from build123d import *

# Parameters (mm, degrees)
F0_W     = 25.908
F0_H     = 5.08
F1_DEPTH = 3.048
F2_W     = 25.908
F2_H     = 3.048
F3_DEPTH = 28.448
F4_R     = 0.762
F4_R_2   = 1.27
F5_DEPTH = 25.4
F6_R     = 1.778
F7_DEPTH = 25.4
F8_DEPTH = 2.032


with BuildPart() as f1:
    # F0 (on Top) → F1 (new body)
    with BuildSketch(Plane.XY):
        Rectangle(F0_W, F0_H)
    extrude(amount=F1_DEPTH)

    # F2 (on face) → F3 (join)
    with BuildSketch(Plane(origin=(0, 0, 0), x_dir=(1, 0, 0), z_dir=(0, 0, -1))):
        with Locations((0, 4.064)):
            Rectangle(F2_W, F2_H)
    extrude(amount=-F3_DEPTH)

    # F4 (on face) → F5 (cut)
    with BuildSketch(Plane.XZ.offset(5.588)):
        with Locations((-8.128, 14.224)):
            Circle(F4_R)
        with Locations((-8.128, 17.78)):
            Circle(F4_R)
        with Locations((-8.128, 10.668)):
            Circle(F4_R)
        with Locations((-3.556, 6.096)):
            Circle(F4_R)
        with Locations((0, 6.096)):
            Circle(F4_R)
        with Locations((3.556, 6.096)):
            Circle(F4_R)
        with Locations((8.128, 10.668)):
            Circle(F4_R)
        with Locations((8.128, 14.224)):
            Circle(F4_R)
        with Locations((8.128, 17.78)):
            Circle(F4_R)
        with Locations((3.556, 22.352)):
            Circle(F4_R)
        with Locations((0, 22.352)):
            Circle(F4_R)
        with Locations((-3.556, 22.352)):
            Circle(F4_R)
        with Locations((0, 14.224)):
            Circle(F4_R_2)
    extrude(amount=-F5_DEPTH, mode=Mode.SUBTRACT)

    # F6 (on face) → F7 (cut)
    with BuildSketch(Plane.XY.offset(3.048)):
        with Locations((-9.652, 0)):
            Circle(F6_R)
        Circle(F6_R)
        with Locations((9.652, 0)):
            Circle(F6_R)
    extrude(amount=-F7_DEPTH, mode=Mode.SUBTRACT)

    # F8 (add): a face of the model
    f8_faces = [f1.faces().sort_by_distance(p)[0] for p in [
        (0, 2.2684693667, 0),
    ]]
    extrude(f8_faces, amount=F8_DEPTH)


solid = f1.part
The listing builds one solid part. Answer for the finished solid, in the listing's coordinates (mm). A direction names the side the tool comes from. Coordinates: 2 decimals unless noted, no trailing zeros. Loops run counter-clockwise (first coordinate to the right, second up) from the corner with the lowest first, then second, coordinate; pieces in that order, holes last. Notation, with made-up numbers: M 85,76 L 135,76 A24 ccw 135,114 Z; hole C -17,-35.5 d6. An arc over 180 degrees is marked long. Answer in a Markdown table with one row per item.
1) Find the intervals of material crossed by probe 1 along Z at (x, y) = (0.5, -4.5); probe 2 along Y at (x, z) = (2, 11.5); probe 3 along X at (y, z) = (-3.5, 22), in increasing order.
Answers below:
| item | result |
|---|---|
| probe 1 | -2.03 to 5.52, 6.67 to 13.06, 15.39 to 21.78, 22.93 to 28.45 |
| probe 2 | -5.59 to -2.54 |
| probe 3 | -12.95 to -4.23, -2.88 to -0.68, 0.68 to 2.88, 4.23 to 12.95 |
2) Find section C-C (z = 17.78). Determine the outline of the cut face in (x, y).
Answers below:
| item | result |
|---|---|
| outline | M -12.95,-5.59 L -8.89,-5.59 L -8.89,-2.54 L -12.95,-2.54 Z; M -7.37,-5.59 L 7.37,-5.59 L 7.37,-2.54 L -7.37,-2.54 Z; M 8.89,-5.59 L 12.95,-5.59 L 12.95,-2.54 L 8.89,-2.54 Z |
3) Given pin 1 (2 mm diameter, centred on x = -8, y = 0.5, fed in from +Z); pin 2 (4 mm diameter, centred on x = 5.5, z = 22, fed in from +Y); pin 3 (0.9 mm diameter, centred on x = -8.128, z = 14.224, fed in from +Y), each flat-ended and moving along its own axis, determine where each tip first touches the part or whether it passes through.
Answers below:
| item | result |
|---|---|
| pin 1 | z = 3.05 |
| pin 2 | y = -2.54 |
| pin 3 | through |
4) Determine the mould class of faces 3 (the flat face through (0, -2, -2.032)), 4 (the cylindrical face through (-0.385, -1.736, 0.544)), 5 (the flat face through (12.954, -3, 10)) for opening direction X: released by +X, released by -X, zero draft, split by the parting line, or undercut.
Answers below:
| item | result |
|---|---|
| face 3 | zero draft |
| face 4 | undercut |
| face 5 | released by +X |
5) Find section B-B (y = 0). Determine the outline of the cut face in (x, z).
Answers below:
| item | result |
|---|---|
| outline | M -12.95,-2.03 L -11.43,-2.03 L -11.43,3.05 L -12.95,3.05 Z; M -7.87,-2.03 L -1.78,-2.03 L -1.78,3.05 L -7.87,3.05 Z; M 1.78,-2.03 L 7.87,-2.03 L 7.87,3.05 L 1.78,3.05 Z; M 11.43,-2.03 L 12.95,-2.03 L 12.95,3.05 L 11.43,3.05 Z |
6) Find section D-D (z = 0.5). Determine the outline of the cut face in (x, y).
Answers below:
| item | result |
|---|---|
| outline | M -12.95,-5.59 L 12.95,-5.59 L 12.95,2.54 L -12.95,2.54 Z; hole C -9.65,0 d3.56; hole C 0,0 d3.56; hole C 9.65,0 d3.56 |
7) Which of the six approach directions +Z, -Z, +X, -X, +Y, -Y give full straight-line access (tool end or side, diameter ignored) to faces 1 (the flat face through (0, 2, 3.048)), 2 (the flat face through (0, 2.54, 1))?
Answers below:
| item | result |
|---|---|
| face 1 | +Z, +X, -X, +Y |
| face 2 | +Z, -Z, +X, -X, +Y |
8) Find section A-A (x = 0). Determine the outline of the cut face in (y, z).
Answers below:
| item | result |
|---|---|
| outline | M -5.59,-2.03 L -1.78,-2.03 L -1.78,3.05 L -2.54,3.05 L -2.54,5.33 L -5.59,5.33 Z; M -5.59,6.86 L -2.54,6.86 L -2.54,12.95 L -5.59,12.95 Z; M -5.59,15.49 L -2.54,15.49 L -2.54,21.59 L -5.59,21.59 Z; M -5.59,23.11 L -2.54,23.11 L -2.54,28.45 L -5.59,28.45 Z; M 1.78,-2.03 L 2.54,-2.03 L 2.54,3.05 L 1.78,3.05 Z |
